from build123d import *

# Parameters (mm, degrees)
BOSS_EXTRUDE1_DEPTH            = 1.6
F_3_2_3_2_DIAMETER_HOLE1_D     = 3.2
F_3_2_3_2_DIAMETER_HOLE1_DEPTH = 4
F_3_2_3_2_DIAMETER_HOLE1_TIP   = 0.96137699
SKETCH8_R                      = 1.6
CUT_EXTRUDE2_DEPTH             = 205.459189082


with BuildPart() as part:
    # Sketch1 → Boss-Extrude1 (new body)
    with BuildSketch(Plane.XY):
        Polygon((0, 0), (140, 0), (140, 44), (149, 44), (149, 96), (140, 96), (140, 140), (0, 140), (0, 96), (-9, 96), (-9, 44), (0, 44), align=None)
    extrude(amount=BOSS_EXTRUDE1_DEPTH)

    # Ø3.2 (3.2) Diameter Hole1
    with Locations(Plane(origin=(0, 0, 0), x_dir=(-1, 0, 0), z_dir=(0, 0, -1))):
        with Locations((-130, 92), (-130, 48), (-10, 92), (-10, 48)):
            Hole(F_3_2_3_2_DIAMETER_HOLE1_D / 2, depth=F_3_2_3_2_DIAMETER_HOLE1_DEPTH)
            with Locations((0, 0, -(F_3_2_3_2_DIAMETER_HOLE1_DEPTH + F_3_2_3_2_DIAMETER_HOLE1_TIP / 2))):  # 118° drill point
                Cone(0, F_3_2_3_2_DIAMETER_HOLE1_D / 2, F_3_2_3_2_DIAMETER_HOLE1_TIP, mode=Mode.SUBTRACT)

    # Sketch8 → Cut-Extrude2 (cut, through all)
    with BuildSketch(Plane.XY.offset(1.6)):
        with Locations((-5, 92)):
            Circle(SKETCH8_R)
        with Locations((-5, 48)):
            Circle(SKETCH8_R)
        with Locations((145, 70)):
            Circle(SKETCH8_R)
    extrude(amount=-CUT_EXTRUDE2_DEPTH, mode=Mode.SUBTRACT)


solid = part.part
Geometry check sheet. Reference: the model listing, model coordinates, mm. Round coordinates to 2 decimals unless told otherwise and drop trailing zeros. Write each loop counter-clockwise with the first axis right and the second up, starting at its lowest first coordinate (ties: lowest second). Pieces come first, ordered by that corner, then holes. Notation, with made-up numbers: (59.25, 22.5) - (97.25, 22.5) arc R25 ccw to (97.25, 47.5) - close; hole circle Ø1 at (-17, -27). An arc over 180 degrees is marked (long way). One line per item, written item: value.
1. Mould release check, pull along Y, two halves, no side actions. Record for faces 1 (the face through (8.4, 92.07, 0.81)), 2 (the face through (69, 71, 1.6)), 3 (the face through (-5.208, 93.586, 0.811)): released by +Y, released by -Y, zero draft, split by the parting line, or undercut.
The answers:
face 1: undercut
face 2: zero draft
face 3: undercut
2. Scan lines: L1, parallel to X at y = 92, z = 1.05; L2, parallel to Y at x = 130, z = 0.75; L3, parallel to X at y = 18, z = 0.7. Record each from-to range of solid material in increasing order.
The answers:
L1: x = -9 to -6.6, -3.4 to 8.4, 11.6 to 128.4, 131.6 to 149
L2: y = 0 to 46.4, 49.6 to 90.4, 93.6 to 140
L3: x = 0 to 140
3. Cross-section at B-B on y = 9.5. Record the boundary of the cut face in (x, z).
The answers:
outline: (0, 0) - (140, 0) - (140, 1.6) - (0, 1.6) - close
4. Cross-section at A-A on z = 0.4. Record the boundary of the cut face in (x, y).
The answers:
outline: (-9, 44) - (0, 44) - (0, 0) - (140, 0) - (140, 44) - (149, 44) - (149, 96) - (140, 96) - (140, 140) - (0, 140) - (0, 96) - (-9, 96) - close; hole circle Ø3.2 at (-5, 48); hole circle Ø3.2 at (-5, 92); hole circle Ø3.2 at (10, 48); hole circle Ø3.2 at (10, 92); hole circle Ø3.2 at (130, 48); hole circle Ø3.2 at (130, 92); hole circle Ø3.2 at (145, 70)
5. Depth check by flat-ended pin: pin 1 Ø0.8 at (y, z) = (12.5, 1) entering from +X; pin 2 Ø0.8 at (y, z) = (128.5, 0.5) entering from -X; pin 3 Ø0.5 at (x, z) = (146.5, 0.5) entering from +Y. Enter the tip coordinate at first touch or a pass-through.
The answers:
pin 1: stops at x = 140
pin 2: stops at x = 0
pin 3: stops at y = 96
